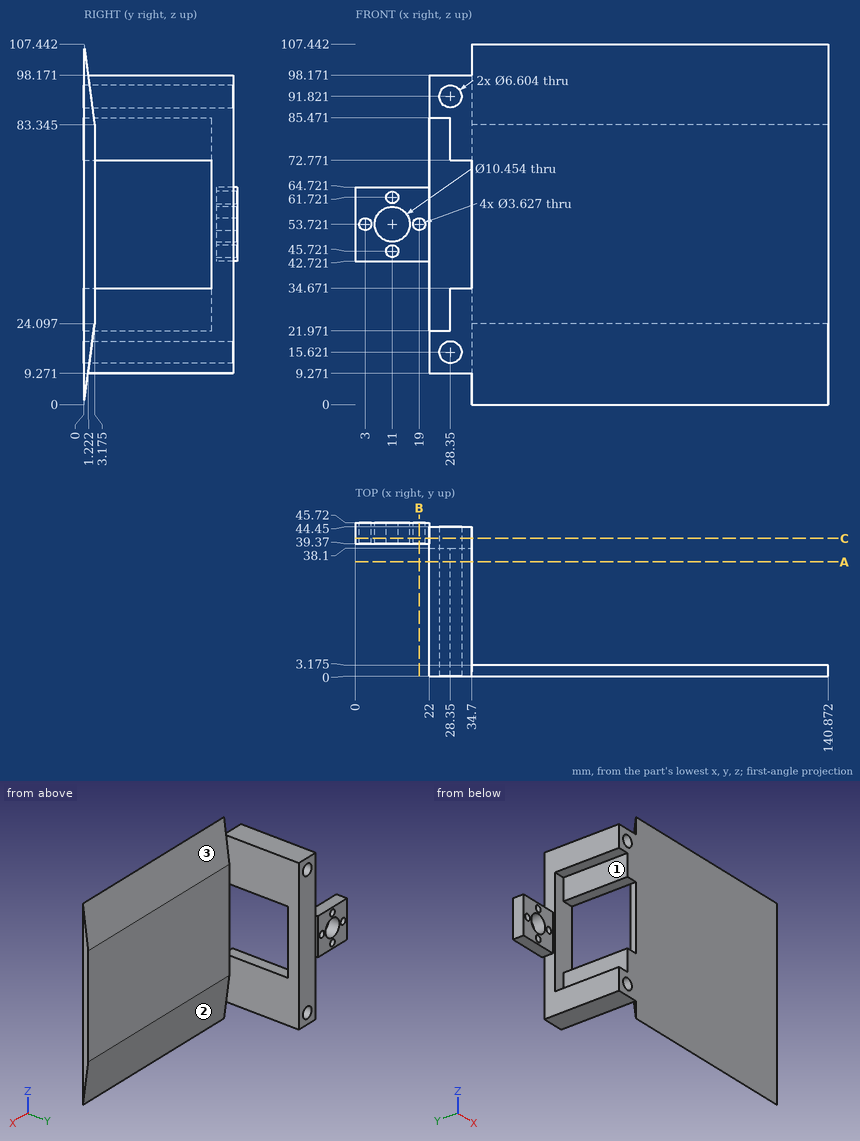
Part print with two shaded views. Sizes in mm from the minimum x, y, z corner. A direction names the side the tool comes from. Give positions to 0.01 mm unless a question says otherwise; leave off trailing zeros. Order: outer loops, then holes, each group sorted by start corner. A loop starts at its lowest first (then second) coordinate and runs counter-clockwise, first axis right, second up.
1) Saw through at A-A, the plane y = 34. Write the cut outline in (x, z).
2) Saw through at C-C, the plane y = 41. Count the separate pieces of the cut face and the enclosed holes in it, then the cut area to 3 significant figures.
3) Wall check: probe 1 along Z at (x, y) = (11, 43) (1 decimal); probe 2 along Z at (x, y) = (3, 43) (1 decimal); probe 3 along X at (y, z) = (31, 25.5). Give the ranges that are in metal, low to high.
4) 3-axis set-ups, long thin cutter, end or side, ignore diameter. For the marked faces 1, 2 and 3: which of +Z, -Z, +X, -X, +Y, -Y reach the whole face in a straight line?
5) Pin check, flat tips, straight feed: pin 1 (12 mm diameter, centred on y = 35, z = 13, fed in from +X); pin 2 (0.6 mm diameter, centred on y = 0.5, z = 104, fed in from -X); pin 3 (7 mm diameter, centred on x = 10.5, y = 41.5, fed in from +Z). Stop position of each tip, or through.
6) Saw through at B-B, the plane x = 19. Write the cut outline in (y, z) (1 decimal), then the cut area to 3 significant figures.
Computed:
1. outline: (22, 9.27) - (34.7, 9.27) - (34.7, 34.67) - (28.35, 34.67) - (28.35, 21.97) - (22, 21.97) - close; (22, 85.47) - (28.35, 85.47) - (28.35, 72.77) - (34.7, 72.77) - (34.7, 98.17) - (22, 98.17) - close; hole circle Ø6.6 at (28.35, 15.62); hole circle Ø6.6 at (28.35, 91.82)
2. separate pieces: 1
2. enclosed holes: 7
2. area: 1,420 mm2
3. probe 1: z = 42.7 to 43.9, 47.5 to 48.5, 58.9 to 59.9, 63.5 to 64.7
3. probe 2: z = 42.7 to 51.9, 55.5 to 64.7
3. probe 3: x = 28.35 to 34.7
4. face 1: -X, -Y
4. face 2: -Z, +X, +Y
4. face 3: +Z, +X, +Y
5. pin 1: stops at x = 34.7
5. pin 2: stops at x = 34.7
5. pin 3: stops at z = 64.72
6. outline: (39.4, 42.7) - (45.7, 42.7) - (45.7, 51.9) - (39.4, 51.9) - close; (39.4, 55.5) - (45.7, 55.5) - (45.7, 64.7) - (39.4, 64.7) - close
6. area: 117 mm2
